Autodesk Inventor part; units mm, degrees
ref_plane "YZ Plane" through (0, 0, 0) normal (1, 0, 0) x (0, 1, 0)
ref_plane "XZ Plane" through (0, 0, 0) normal (0, 1, 0) x (-1, 0, 0)
ref_plane "XY Plane" through (0, 0, 0) normal (0, 0, 1) x (1, 0, 0)
ref_plane "Work Plane1" through (0, 0, -14.5) normal (0, 0, 1) x (1, 0, 0)
sketch "Sketch1" plane through (0, 0, -14.5) normal (0, 0, 1) x (1, 0, 0)
  arc A0 (10.3187, 25) -> (15, 22.0046) centre (12.05, 22.55) ccw
  line L0 (15, 22.0046) -> (15, 25)
  line L1 (15, 25) -> (10.3187, 25)
  circle A1 centre (12.05, 22.55) radius 1.45
  arc A2 (15, -22.0046) -> (10.3187, -25) centre (12.05, -22.55) ccw
  line L2 (10.3187, -25) -> (15, -25)
  line L3 (15, -25) -> (15, -22.0046)
  circle A3 centre (12.05, -22.55) radius 1.45
  arc A4 (-10.3187, -25) -> (-15, -22.0046) centre (-12.05, -22.55) ccw
  line L4 (-15, -22.0046) -> (-15, -25)
  line L5 (-15, -25) -> (-10.3187, -25)
  circle A5 centre (-12.05, -22.55) radius 1.45
  circle A6 centre (-12.05, 22.55) radius 1.45
  arc A7 (-15, 22.0046) -> (-10.3187, 25) centre (-12.05, 22.55) ccw
  line L6 (-10.3187, 25) -> (-15, 25)
  line L7 (-15, 25) -> (-15, 22.0046)
  point P0 (0, 0)
extrude "Extrusion1" add sketch "Sketch1" along normal blind 15
sketch "Sketch2" plane through (0, 0, 0.5) normal (0, 0, 1) x (1, 0, 0)
  line L0 (15, 22.0046) -> (15, 25)
  line L1 (15, 25) -> (10.3187, 25)
  arc A0 (10.3187, 25) -> (15, 22.0046) centre (12.05, 22.55) ccw
  circle A1 centre (12.05, 22.55) radius 1.45
  line L2 (10.3187, -25) -> (15, -25)
  line L3 (15, -25) -> (15, -22.0046)
  arc A2 (15, -22.0046) -> (10.3187, -25) centre (12.05, -22.55) ccw
  circle A3 centre (12.05, -22.55) radius 1.45
  line L4 (-15, -22.0046) -> (-15, -25)
  line L5 (-15, -25) -> (-10.3187, -25)
  arc A4 (-10.3187, -25) -> (-15, -22.0046) centre (-12.05, -22.55) ccw
  circle A5 centre (-12.05, -22.55) radius 1.45
  line L6 (-10.3187, 25) -> (-15, 25)
  line L7 (-15, 25) -> (-15, 22.0046)
  arc A6 (-15, 22.0046) -> (-10.3187, 25) centre (-12.05, 22.55) ccw
  circle A7 centre (-12.05, 22.55) radius 1.45
  line L8 (15, 25) -> (10.3187, 25)
  line L9 (-15, -25) -> (-10.3187, -25)
  line L10 (15, 25) -> (-15, 25)
  line L11 (-15, 25) -> (-15, -25)
  line L12 (-15, -25) -> (15, -25)
  line L13 (15, -25) -> (15, 25)
  point P0 (0, 0)
extrude "Extrusion2" add sketch "Sketch2" along normal blind 2 contours A0 L1 L0 | L13 A2 L12 A4 L11 A6 L10 A0 | L3 L2 A2 | A6 L7 L6 | L5 L4 A4 | A1 | A3 | A5 | A7
sketch "Sketch3" plane through (0, 0, -14.5) normal (0, 0, -1) x (-1, 0, 0)
  circle A0 centre (12.05, 22.55) radius 1.45
  circle A1 centre (-12.05, 22.55) radius 1.45
  circle A2 centre (-12.05, -22.55) radius 1.45
  circle A3 centre (12.05, -22.55) radius 1.45
  line L0 (15, -25) -> (-15, -25)
  line L1 (15, 25) -> (15, -25)
  line L2 (-15, 25) -> (15, 25)
  line L3 (-15, -25) -> (-15, 25)
  circle A4 centre (12.05, -22.55) radius 1.45
  circle A5 centre (-12.05, -22.55) radius 1.45
  circle A6 centre (-12.05, 22.55) radius 1.45
  circle A7 centre (12.05, 22.55) radius 1.45
  point P0 (0, 0)
hole "Hole1" at (-12.05, -22.55, -14.5) at (12.05, -22.55, -14.5) at (12.05, 22.55, -14.5) at (-12.05, 22.55, -14.5) direction (0, 0, 1) diameter 4 depth 5 counterbore diameter 4.5 counterbore depth 0.5
sketch "Sketch4" plane through (0, 0, 0.5) normal (0, 0, -1) x (-1, 0, 0)
  circle A0 centre (12.05, 22.55) radius 1.45
  circle A1 centre (-12.05, 22.55) radius 1.45
  circle A2 centre (-12.05, -22.55) radius 1.45
  circle A3 centre (12.05, -22.55) radius 1.45
  line L0 (15, -25) -> (-15, -25)
  line L1 (15, 25) -> (15, -25)
  line L2 (-15, 25) -> (15, 25)
  line L3 (-15, -25) -> (-15, 25)
  line L4 (0, 12.5) -> (0, -12.5)
  point P0 (0, 0)
  dimension "d11" = 12.5
  dimension "d12" = 12.5
  dimension "d13" = 12.5
  dimension "d14" = 12.5
hole "Hole2" at (0, 12.5, 0.5) at (0, -12.5, 0.5) direction (0, 0, 1) diameter 3.4 depth 5 countersink diameter 7 countersink angle 90
equation "\"d11\" = d12"
properties part number "buck_holder" material "Glass"
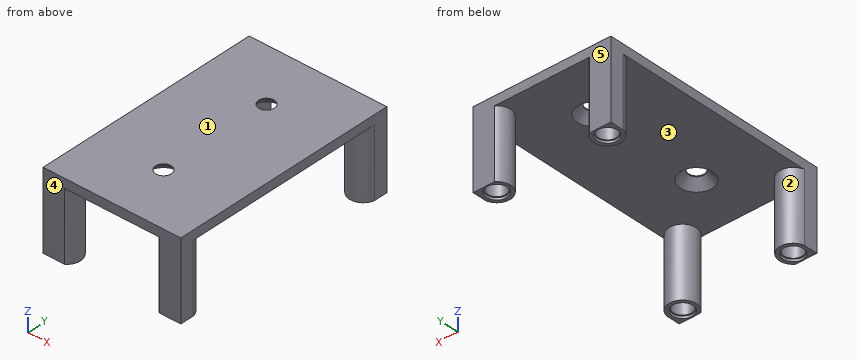
Design review of the part built by this model. Coordinates are the model's own, in mm. Face numbers are marked on the shaded views. A direction names the side the tool comes from. Coordinates: 2 decimals unless noted, no trailing zeros. Order: outer loops, then holes, each group sorted by start corner. A loop starts at its lowest first (then second) coordinate and runs counter-clockwise, first axis right, second up. Notation, with made-up numbers: (-14, 75) -> (28, 75) arc R17 cw to (28, 87) -> close; hole circle Ø10 at (-28, -20). An arc over 180 degrees is marked (long way). One line per item, written item: value. Start each with the question number.
Q1. Insertion check: pin 1 Ø3 at (x, y) = (0, -12.5) entering from +Z; pin 2 Ø3.5 at (x, y) = (12.05, -22.55) entering from -Z; pin 3 Ø1.4 at (x, y) = (11.5, -22.5) entering from -Z; pin 4 Ø3 at (x, y) = (-11.5, 23) entering from -Z. Each pin has a flat end and moves straight along its axis. Give the tip position at first contact, or say it passes through.
Q2. Take a section at A-A, the plane y = 12.5. State the section outline as (x, z) points, then the cut area to 3 significant figures.
Q3. Mouldability with a two-part tool opening along Y and no side actions: class the marked faces 3, 4 and 5 as pulls with the +Y half, pulls with the -Y half, needs draft (parallel to the pull), parting line crosses it, or undercut.
Q4. For probe 1 along Y at (x, z) = (12.05, -14.3); probe 2 along Y at (x, z) = (12.05, -6.5); probe 3 along X at (y, z) = (22.55, -12.8), list the stretches that pass through material, from the lowest coordinate up.
Q5. Tool access review of the marked faces 1 and 2: name each direction out of +Z, -Z, +X, -X, +Y, -Y from which nothing blocks a thin tool from reaching the whole face with its end or side.
Q6. Take a section at B-B, the plane z = -2. State the section outline as (x, y) points, then the cut area to 3 significant figures.
Values follow:
1. pin 1: passes through
1. pin 2: stops at z = -9.5
1. pin 3: stops at z = 0.5
1. pin 4: stops at z = -14
2. outline: (-15, 0.5) -> (-3.5, 0.5) -> (-1.7, 2.3) -> (-1.7, 2.5) -> (-15, 2.5) -> close; (1.7, 2.3) -> (3.5, 0.5) -> (15, 0.5) -> (15, 2.5) -> (1.7, 2.5) -> close
2. area: 50.0 mm2
3. face 3: undercut
3. face 4: pulls with the -Y half
3. face 5: pulls with the +Y half
4. probe 1: y = -25 to -24.8, -20.3 to -19.55, 19.55 to 20.3, 24.8 to 25
4. probe 2: y = -25 to -24, -21.1 to -19.55, 19.55 to 21.1, 24 to 25
4. probe 3: x = -15 to -14.05, -10.05 to -9.05, 9.05 to 10.05, 14.05 to 15
5. face 1: +Z, +X, -X, +Y, -Y
5. face 2: -Z
6. outline: (-15, -25) -> (-10.32, -25) arc R3 ccw (long way) to (-15, -22) -> close; (-15, 22) arc R3 ccw (long way) to (-10.32, 25) -> (-15, 25) -> close; (10.32, -25) -> (15, -25) -> (15, -22) arc R3 ccw (long way) to start; (10.32, 25) arc R3 ccw (long way) to (15, 22) -> (15, 25) -> close; hole circle Ø2.9 at (-12.05, -22.55); hole circle Ø2.9 at (-12.05, 22.55); hole circle Ø2.9 at (12.05, -22.55); hole circle Ø2.9 at (12.05, 22.55)
6. area: 84.6 mm2
